from build123d import *

# Parameters (mm, degrees)
F0_R     = 15.875
F0_W     = 78.74
F0_H     = 53.34
F1_DEPTH = 12.7


with BuildPart() as f1:
    # F0 (on Front) → F1 (new body)
    with BuildSketch(Plane.XZ):
        with BuildLine():
            Line((-22.039405, 0), (22.039405, 0))
            ThreePointArc((22.039405, 0), (107.95, 66.04), (193.860595, 0))
            Line((193.860595, 0), (222.25, 0))
            Line((222.25, 0), (222.25, 152.4))
            Line((222.25, 152.4), (196.85, 152.4))
            Line((196.85, 152.4), (196.85, 155.575))
            Line((196.85, 155.575), (219.075, 155.575))
            Line((219.075, 155.575), (219.075, 200.025))
            Line((219.075, 200.025), (196.85, 200.025))
            Line((196.85, 200.025), (196.85, 203.2))
            Line((196.85, 203.2), (-196.85, 203.2))
            Line((-196.85, 203.2), (-196.85, 200.025))
            Line((-196.85, 200.025), (-219.075, 200.025))
            Line((-219.075, 200.025), (-219.075, 155.575))
            Line((-219.075, 155.575), (-196.85, 155.575))
            Line((-196.85, 155.575), (-196.85, 152.4))
            Line((-196.85, 152.4), (-222.25, 152.4))
            Line((-222.25, 152.4), (-222.25, 0))
            Line((-222.25, 0), (-193.860595, 0))
            ThreePointArc((-193.860595, 0), (-107.95, 66.04), (-22.039405, 0))
        make_face()
        with Locations((-165.1, 99.06)):
            Circle(F0_R, mode=Mode.SUBTRACT)
        with Locations((-82.55, 99.06)):
            Circle(F0_R, mode=Mode.SUBTRACT)
        with Locations((0, 99.06)):
            Circle(F0_R, mode=Mode.SUBTRACT)
        with Locations((82.55, 99.06)):
            Circle(F0_R, mode=Mode.SUBTRACT)
        with Locations((165.1, 99.06)):
            Circle(F0_R, mode=Mode.SUBTRACT)
        with Locations((-119.38, 157.48)):
            Rectangle(F0_W, F0_H, mode=Mode.SUBTRACT)
        with Locations((0, 157.48)):
            Rectangle(F0_W, F0_H, mode=Mode.SUBTRACT)
        with Locations((119.38, 157.48)):
            Rectangle(F0_W, F0_H, mode=Mode.SUBTRACT)
    extrude(amount=F1_DEPTH)


solid = f1.part
CAD build for the part. Positions are in the model's coordinates, mm. A direction names the side the tool comes from. Give positions to 0.01 mm unless a question says otherwise; leave off trailing zeros. Write each loop counter-clockwise with the first axis right and the second up, starting at its lowest first coordinate (ties: lowest second). Pieces come first, ordered by that corner, then holes. Notation, with made-up numbers: M 49,-1 L 83,-1 A20 cw 83,28 Z; hole C 61.25,82.25 d2. An arc over 180 degrees is marked long. Put each result on its own line as item: value. Start each with the question number.
(1) Flat gauge pins, fed straight in: pin 1 Ø5 at (x, y) = (-65, -4) entering from -Z; pin 2 Ø2.5 at (y, z) = (-5, 154) entering from +X; pin 3 Ø19 at (x, z) = (82.55, 99.06) entering from +Y; pin 4 Ø1 at (y, z) = (-8.5, 201.5) entering from -X. Where does each tip first touch, or does it go through?
(2) Band-saw the part on B-B, the plane z = 99.06. Write the cut outline in (x, y) (3 decimals).
(3) Band-saw the part on D-D, the plane z = 16.5. Write the cut outline in (x, y), and give its area (3 significant figures).
(4) Mould opens along X. For faces 1 (the face through (-39.37, -6, 157)), 2 (the face through (-208, -6, 0)), 3 (the face through (-222.25, -6, 77)) say: +X half, -X half, draft (parallel to the pull), parting line (faces both ways), or undercut.
(5) Probe L1, parallel to X at y = -8.25, z = 143; L2, parallel to Z at x = 82.55, y = -7.5 (3 decimals); L3, parallel to X at y = -7.25, z = 84.5. List the from-to ranges inside material, lowest first.
(6) Which spindle directions (+Z, -Z, +X, -X, +Y, -Y) get a long thin tool onto all of the face, cutting with end or side? Do faces 4 (the face through (208, -6, 200.025)), 5 (the face through (208, -6, 155.575)), 6 (the face through (-120, -6, 184.15)). Say none if no direction does.
(7) Band-saw the part on A-A, the plane x = 0. Write the cut outline in (y, z) (3 decimals).
(8) Band-saw the part on C-C, the plane x = -165.1. Write the cut outline in (y, z) (3 decimals), and give its area (3 significant figures).
Response values:
1. pin 1: stops at z = 53.54
1. pin 2: stops at x = 196.85
1. pin 3: passes through
1. pin 4: stops at x = -196.85
2. outline: M -222.25,-12.7 L -180.975,-12.7 L -180.975,0 L -222.25,0 Z; M -149.225,-12.7 L -98.425,-12.7 L -98.425,0 L -149.225,0 Z; M -66.675,-12.7 L -15.875,-12.7 L -15.875,0 L -66.675,0 Z; M 15.875,-12.7 L 66.675,-12.7 L 66.675,0 L 15.875,0 Z; M 98.425,-12.7 L 149.225,-12.7 L 149.225,0 L 98.425,0 Z; M 180.975,-12.7 L 222.25,-12.7 L 222.25,0 L 180.975,0 Z
3. outline: M -222.25,-12.7 L -187.66,-12.7 L -187.66,0 L -222.25,0 Z; M -28.24,-12.7 L 28.24,-12.7 L 28.24,0 L -28.24,0 Z; M 187.66,-12.7 L 222.25,-12.7 L 222.25,0 L 187.66,0 Z
3. area: 1,600 mm2
4. face 1: undercut
4. face 2: draft
4. face 3: -X half
5. L1: x = -222.25 to -158.75, -80.01 to -39.37, 39.37 to 80.01, 158.75 to 222.25
5. L2: z = 62.334 to 83.185, 114.935 to 130.81, 184.15 to 203.2
5. L3: x = -222.25 to -171.43, -158.77 to -88.88, -76.22 to -6.33, 6.33 to 76.22, 88.88 to 158.77, 171.43 to 222.25
6. face 4: +Z, +X, +Y, -Y
6. face 5: +X, +Y, -Y
6. face 6: +Y, -Y
7. outline: M -12.7,0 L 0,0 L 0,83.185 L -12.7,83.185 Z; M -12.7,114.935 L 0,114.935 L 0,130.81 L -12.7,130.81 Z; M -12.7,184.15 L 0,184.15 L 0,203.2 L -12.7,203.2 Z
8. outline: M -12.7,45.236 L 0,45.236 L 0,83.185 L -12.7,83.185 Z; M -12.7,114.935 L 0,114.935 L 0,203.2 L -12.7,203.2 Z
8. area: 1,600 mm2
